Can you work these out from the model? Positions are in its coordinate system, mm. A direction names the side the tool comes from. Give positions to 0.01 mm unless a question says otherwise; leave off trailing zeros. Write each loop counter-clockwise with the first axis right and the second up, starting at its lowest first coordinate (ties: lowest second). Pieces come first, ordered by that corner, then holes.
from build123d import *

# Parameters (mm, degrees)
SKETCH_1_R           = 12.5
SKETCH_1_R_2         = 5
EXTRUDE_1_DEPTH      = 15
SKETCH_1_3_R         = 5
EXTRUDE_2_DEPTH      = 10
EXTRUDE_3_REACH      = 165.669
EXTRUDE_3_END_RADIUS = 12.5
SKETCH_2_R           = 5


with BuildPart() as part:
    # Sketch 1 → Extrude 1 (new body)
    with BuildSketch(Plane(origin=(0, 0, 0), x_dir=(0, 0, -1), z_dir=(1, 0, 0))):
        Circle(SKETCH_1_R)
        Circle(SKETCH_1_R_2, mode=Mode.SUBTRACT)
        Circle(SKETCH_1_R_2)
    extrude(amount=EXTRUDE_1_DEPTH)

    # Sketch 1_3 → Extrude 2 (add)
    with BuildSketch(Plane(origin=(0, 0, 0), x_dir=(0, 0, -1), z_dir=(1, 0, 0))):
        Circle(SKETCH_1_3_R)
    extrude(amount=-EXTRUDE_2_DEPTH)

    # Extrude 3: up to this cylinder (the profile starts outside it)
    extrude_3_end = Plane(origin=(7.5, 0, 0), z_dir=(-1, 0, 0)) * Cylinder(EXTRUDE_3_END_RADIUS, 357.338, mode=Mode.PRIVATE)
    # Sketch 2 → Extrude 3 (add, up to the surface)
    with BuildSketch(Plane(origin=(0, 150, 0), x_dir=(1, 0, 0), z_dir=(0, 1, 0)), mode=Mode.PRIVATE) as extrude_3_sk1:
        with Locations(Location((7.5, 0, 0), (0, 0, 270))):
            Circle(SKETCH_2_R)
    extrude_3_tool1 = extrude(extrude_3_sk1.sketch, amount=-EXTRUDE_3_REACH, mode=Mode.PRIVATE) - extrude_3_end
    add(extrude_3_tool1.solids().sort_by_distance((7.5, 150, 0))[0])


solid = part.part
(1) Imagine slicing it at B-B, the plane y = 0. Write out the boundary of the cut face in (x, z), plus the area to 3 significant figures.
Returned:
outline: (-10, -5) - (0, -5) - (0, -12.5) - (15, -12.5) - (15, 12.5) - (0, 12.5) - (0, 5) - (-10, 5) - close
area: 475 mm2
(2) If I drill on L1, parallel to Y at x = 4.25, z = -0.25; L2, parallel to Z at x = 8, y = 102; L3, parallel to Y at x = 11, z = -10.75, over which ranges is the centre line in solid material (lowest first)?
Returned:
L1: y = -12.5 to 150
L2: z = -4.97 to 4.97
L3: y = -6.38 to 6.38
(3) Imagine slicing it at D-D, the plane y = 37. Write out the boundary of the cut face in (x, z).
Returned:
outline: circle Ø10 at (7.5, 0)
(4) Imagine slicing it at C-C, the plane x = 7.5. Write out the boundary of the cut face in (y, z), plus the area to 3 significant figures.
Returned:
outline: (11.46, -5) - (150, -5) - (150, 5) - (11.46, 5) arc R12.5 ccw (long way) to start
area: 1,870 mm2
(5) Will these pins go through, and if not, where does the flat tip stop? P1, Ø6, axis at x = -5, y = 4.5, coming from the -Z side; P2, Ø10, axis at x = -2.5, z = -9.5, coming from the +Y side; P3, Ø5, axis at x = 1, y = 5, coming from the -Z side.
Returned:
P1: stops at z = -4.77
P2: stops at y = 11.38
P3: stops at z = -12.25
(6) For faces 4 (the face through (0, -5.4, 0.2)), 5 (the face through (15, 0, 0)), which set-ups out of +Z, -Z, +X, -X, +Y, -Y let a thin tool reach every point of the face, with its end or its side?
Returned:
face 4: -X
face 5: +Z, -Z, +X, +Y, -Y
(7) Imagine slicing it at A-A, the plane z = 0. Write out the boundary of the cut face in (x, y).
Returned:
outline: (-10, -5) - (0, -5) - (0, -12.5) - (15, -12.5) - (15, 12.5) - (12.5, 12.5) - (12.5, 150) - (2.5, 150) - (2.5, 12.5) - (0, 12.5) - (0, 5) - (-10, 5) - close
(8) If we mould it in two halves opening along Y, with no side actions, what happens to faces 1 (the face through (-4.93, -4.88, 1.08)), 2 (the face through (12.457, 81.698, -0.651)), 3 (the face through (8, 150, 0))? For each: +Y half, -Y half, draft (parallel to the pull), parting line (faces both ways), or undercut.
Returned:
face 1: parting line
face 2: draft
face 3: +Y half
